For this review, take the finished solid that the model builds, in its own axes (mm). Face numbers are marked on the shaded views. Give positions to 0.01 mm unless a question says otherwise; leave off trailing zeros. Write each loop counter-clockwise with the first axis right and the second up, starting at its lowest first coordinate (ties: lowest second). Pieces come first, ordered by that corner, then holes. Notation, with made-up numbers: M 49,7 L 103,7 A24 cw 103,41 Z; hole C 54.5,-20 d7. An arc over 180 degrees is marked long. Use one line per item in the form item = value. Start each with the question number.
Q1. Mouldability with a two-part tool opening along Y and no side actions: class the marked faces 1 and 2 as released by +Y, released by -Y, zero draft, split by the parting line, or undercut.
Q2. For probe 1 along X at (y, z) = (7.3, -1.05); probe 2 along Y at (x, z) = (-54, 0.45); probe 3 along X at (y, z) = (7.3, -3.45), list the stretches that pass through material, from the lowest coordinate up. Write a range as [from, to].
Q3. Clearance check with flat-ended pins moving along their axes: pin 1 Ø12 at (x, y) = (-31, 46) entering from -Z; pin 2 Ø23.5 at (x, y) = (-41.5, 56.5) entering from -Z. State where each tip first meets the part, or that it passes through.
Q4. Consider section A-A on z = -1.1. Give the number of separate pieces and of enclosed holes in the cut face, and give its area (3 significant figures).
Q5. Consider section B-B on x = -41. Write out the cut boundary in (y, z), and give its area (3 significant figures).
```python
from build123d import *

# Parameters (mm, degrees)
F0_W     = 65.6
F0_H     = 65.6
F0_W_2   = 61.6
F0_H_2   = 61.6
F0_R     = 1.6
F1_DEPTH = 1
F2_DEPTH = 2.91
F3_W     = 4.423
F3_H     = 19.25
F3_W_2   = 6.685
F3_H_2   = 10.487
F3_W_3   = 8
F3_H_3   = 6.25
F3_W_4   = 15.5
F3_W_5   = 13
F3_W_6   = 8.3
F3_H_4   = 3.2
F3_W_7   = 3.35
F3_H_5   = 13.55
F4_DEPTH = 3.911
F5_R     = 1
F6_R     = 2
F7_R     = 3.5
F7_R_2   = 1.6
F8_DEPTH = 4.81
F9_SIZE  = 1


with BuildPart() as f1:
    # F0 (on Top) → F1 (new body)
    with BuildSketch(Plane.XY):
        with Locations((-32.8, 32.8)):
            Rectangle(F0_W, F0_H)
        with Locations((-32.8, 32.8)):
            Rectangle(F0_W_2, F0_H_2, mode=Mode.SUBTRACT)
        with Locations((-32.8, 32.8)):
            Rectangle(F0_W_2, F0_H_2)
        with Locations((-58.3, 7.3)):
            Circle(F0_R, mode=Mode.SUBTRACT)
        with Locations((-7.3, 7.3)):
            Circle(F0_R, mode=Mode.SUBTRACT)
        with Locations((-59.8, 59.8)):
            Circle(F0_R, mode=Mode.SUBTRACT)
        with Locations((-5.8, 59.8)):
            Circle(F0_R, mode=Mode.SUBTRACT)
    extrude(amount=F1_DEPTH)

    # F0 (on Top) → F2 (join)
    with BuildSketch(Plane.XY):
        with Locations((-32.8, 32.8)):
            Rectangle(F0_W, F0_H)
        with Locations((-32.8, 32.8)):
            Rectangle(F0_W_2, F0_H_2, mode=Mode.SUBTRACT)
    extrude(amount=-F2_DEPTH)

    # F3 (on face) → F4 (cut, through all)
    with BuildSketch(Plane.XY.offset(1)):
        with Locations((-63.3885, 26.804)):
            Rectangle(F3_W, F3_H)
        with Locations((-2.2115, 26.804)):
            Rectangle(F3_W, F3_H)
        with Locations((-62.2575, 45.7055)):
            Rectangle(F3_W_2, F3_H_2)
        with Locations((-51.52, 58.912)):
            Rectangle(F3_W_3, F3_H_3)
        with Locations((-35.241, 58.912)):
            Rectangle(F3_W_4, F3_H_3)
        with Locations((-16.462, 58.912)):
            Rectangle(F3_W_5, F3_H_3)
        with Locations((-24.727, 5.641)):
            Rectangle(F3_W_6, F3_H_4)
        with Locations((-8.017, 46.855)):
            Rectangle(F3_W_7, F3_H_5)
    extrude(amount=-F4_DEPTH, mode=Mode.SUBTRACT)

    # F5
    f5_edges = [f1.edges().sort_by_distance(p)[0] for p in [
        (-28.877, 7.241, 0.5),
        (-20.577, 4.041, 0.5),
        (-20.577, 7.241, 0.5),
        (-28.877, 4.041, 0.5),
    ]]
    fillet(f5_edges, radius=F5_R)

    # F6
    f6_edges = [f1.edges().sort_by_distance(p)[0] for p in [
        (-65.6, 0, -0.955),
        (0, 0, -0.955),
        (0, 65.6, -0.955),
        (-65.6, 65.6, -0.955),
    ]]
    fillet(f6_edges, radius=F6_R)

    # F7 (on face) → F8 (join)
    with BuildSketch(Plane(origin=(0, 0, 0), x_dir=(1, 0, 0), z_dir=(0, 0, -1))):
        with Locations((-7.3, -7.3)):
            Circle(F7_R)
        with Locations((-7.3, -7.3)):
            Circle(F7_R_2, mode=Mode.SUBTRACT)
        with Locations((-5.8, -59.8)):
            Circle(F7_R)
        with Locations((-5.8, -59.8)):
            Circle(F7_R_2, mode=Mode.SUBTRACT)
        with Locations((-59.8, -59.8)):
            Circle(F7_R)
        with Locations((-59.8, -59.8)):
            Circle(F7_R_2, mode=Mode.SUBTRACT)
        with Locations((-58.3, -7.3)):
            Circle(F7_R)
        with Locations((-58.3, -7.3)):
            Circle(F7_R_2, mode=Mode.SUBTRACT)
    extrude(amount=F8_DEPTH)

    # F9
    f9_edges = [f1.edges().sort_by_distance(p)[0] for p in [
        (-7.4, 59.8, 1),
        (-8.9, 7.3, 1),
        (-59.9, 7.3, 1),
        (-61.4, 59.8, 1),
    ]]
    chamfer(f9_edges, length=F9_SIZE)


solid = f1.part
```
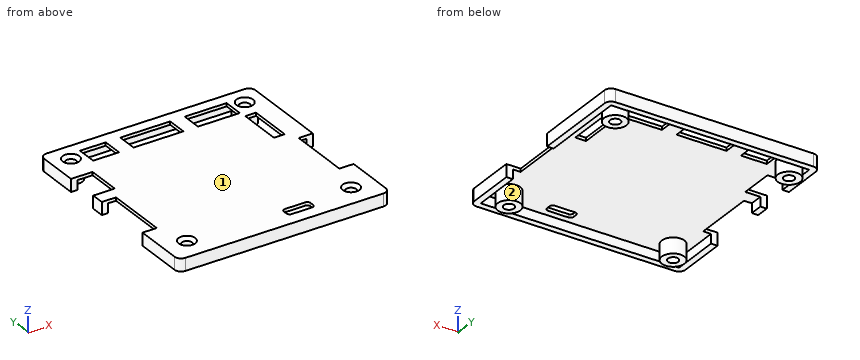
Working result:
q1.face_1 = zero draft
q1.face_2 = undercut
q2.probe_1 = [-65.6, -63.6], [-61.8, -59.9], [-56.7, -54.8], [-10.8, -8.9], [-5.7, -3.8], [-2, 0]
q2.probe_2 = [0, 55.79], [62.04, 65.6]
q2.probe_3 = [-61.8, -59.9], [-56.7, -54.8], [-10.8, -8.9], [-5.7, -3.8]
q3.pin_1 = 0
q3.pin_2 = -2.91
q4.separate_pieces = 7
q4.enclosed_holes = 4
q4.area = 529 mm²
q5.outline = M 0,-2.91 L 2,-2.91 L 2,0 L 55.79,0 L 55.79,1 L 0,1 Z; M 62.04,0 L 63.6,0 L 63.6,-2.91 L 65.6,-2.91 L 65.6,1 L 62.04,1 Z
q5.area = 71.0 mm²
